Could you check a few things on this drawing? It's one solid part, dimensions in mm from its lowest x, y, z. Coordinates: 2 decimals unless noted, no trailing zeros. Order: outer loops, then holes, each group sorted by start corner. A loop starts at its lowest first (then second) coordinate and runs counter-clockwise, first axis right, second up.
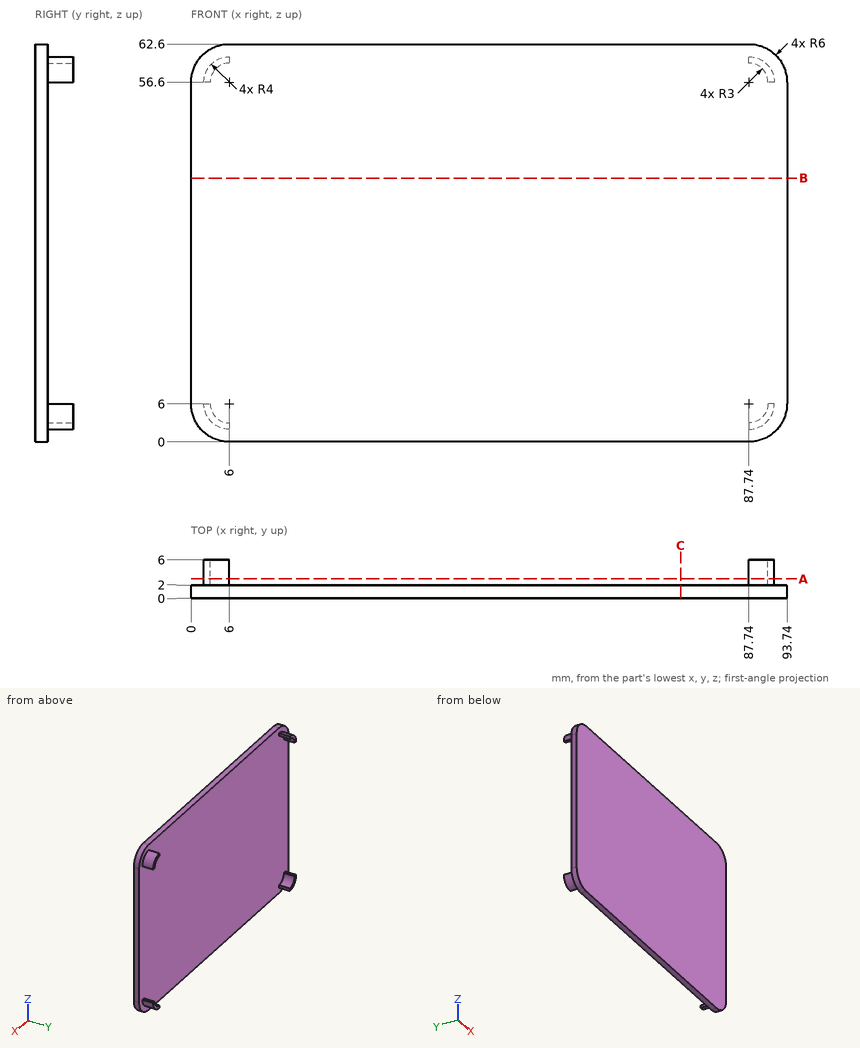
1. I'm going to push flat-ended pins straight in: pin 1 (6 mm diameter, centred on x = 24.5, z = 33, fed in from -Y); pin 2 (1.1 mm diameter, centred on x = 2.5, y = 4, fed in from +Z); pin 3 (0.5 mm diameter, centred on y = 3.5, z = 60, fed in from +X); pin 4 (0.8 mm diameter, centred on y = 3, z = 60, fed in from -X). Where does each tip first touch, or does it pass through?
Completed:
pin 1: stops at y = 0
pin 2: stops at z = 59.3
pin 3: stops at x = 90.21
pin 4: stops at x = 3.35
2. Imagine slicing it at B-B on z = 41.5. Please give me the cut outline in (x, y), then the cut area to 3 significant figures.
Completed:
outline: (0, 0) - (93.74, 0) - (93.74, 2) - (0, 2) - close
area: 187 mm2
3. Imagine slicing it at C-C on x = 77. Please give me the cut outline in (y, z).
Completed:
outline: (0, 0) - (2, 0) - (2, 62.6) - (0, 62.6) - close
4. Please list where this line runs through material, in increasing order: probe 1 along Y at (x, z) = (46.5, 21).
Completed:
probe 1: y = 0 to 2
5. Imagine slicing it at A-A on y = 3. Please give me the cut outline in (x, z).
Completed:
outline: (2, 6) arc R4 ccw to (6, 2) - (6, 3) arc R3 cw to (3, 6) - close; (2, 56.6) - (3, 56.6) arc R3 cw to (6, 59.6) - (6, 60.6) arc R4 ccw to start; (87.74, 2) arc R4 ccw to (91.74, 6) - (90.74, 6) arc R3 cw to (87.74, 3) - close; (87.74, 59.6) arc R3 cw to (90.74, 56.6) - (91.74, 56.6) arc R4 ccw to (87.74, 60.6) - close
